Verification items for the finished model (mm, model axes). A direction names the side the tool comes from. Give positions to 0.01 mm unless a question says otherwise; leave off trailing zeros. Order: outer loops, then holes, each group sorted by start corner. A loop starts at its lowest first (then second) coordinate and runs counter-clockwise, first axis right, second up. Notation, with made-up numbers: (38, -4.5) -> (74, -4.5) arc R20 ccw to (74, 20.5) -> close; hole circle Ø2 at (26, 33). An arc over 180 degrees is marked (long way). Return JSON: item names as keys, results as strings. Group by question number.
(1) Release check for a two-part mould opening along Y. For faces 4 (the face through (-9.2, 0, 10.4)), 5 (the face through (0, 13.4, 12.8)), 6 (the face through (0.046, -17.387, 9.678)), 7 (the face through (0, 12, 6)) record: pulls with the +Y half, pulls with the -Y half, needs draft (parallel to the pull), parting line crosses it, or undercut.
(2) Cross-section at B-B on z = 4. Enter the section's corners in (x, y).
(3) Cross-section at C-C on y = -12.5. Enter the section's corners in (x, z), then the cut area to 3 significant figures.
(4) Depth check by flat-ended pin: pin 1 Ø1.1 at (x, y) = (-12.5, 0) entering from +Z; pin 2 Ø0.8 at (x, y) = (-1, -9) entering from +Z; pin 3 Ø5 at (y, z) = (13.5, 11) entering from -X. Enter the tip coordinate at first touch or a pass-through.
(5) Tool access check on faces 1 (the face through (11, 2.696, 5)), 2 (the face through (11, -2.696, 5)), 3 (the face through (-0.044, 10.565, 8.169)). Record the directions out of +Z, -Z, +X, -X, +Y, -Y that give a thin tool (end or side, any length) a straight path to the whole face; none if there is none.
(6) Cross-section at D-D on z = 7. State how many separate pieces and enclosed holes the cut face has, then the cut area to 3 significant figures.
(7) Thickness scan on line 1 along Y through (x, z) = (2, 9.5); line 2 along X through (y, z) = (1, 6.5); line 3 along Y through (x, z) = (15, 10.25). Record the ranges inside material, lowest first.
(8) Cross-section at A-A on z = 16. Enter the section's corners in (x, y).
from build123d import *

# Parameters (mm, degrees)
F2_R     = 0.5
F3_W     = 21.0270890966
F3_H     = 19.3190067075
F4_DEPTH = 25


with BuildPart() as f1:
    # F0 (on Front) → F1 (revolve)
    with BuildSketch(Plane.XZ):
        with BuildLine():
            Line((-20, 0), (0, 0))
            Line((0, 0), (0, 5))
            add(Edge.make_bspline(
                [(-9, 10.4), (-6.953539399, 4.2876302106), (0, 5)],
                knots=[3.4384028692, 3.4384028692, 3.4384028692, 4.8240705554, 4.8240705554, 4.8240705554], degree=2, weights=[1, 0.7694390741, 1]))
            Line((-9, 10.4), (-9.5, 10.4))
            Line((-9.5, 10.4), (-11.6, 6))
            Line((-11.6, 6), (-13.4, 6))
            Line((-13.4, 6), (-13.4, 20))
            Line((-13.4, 20), (-14.6, 20))
            Line((-14.6, 20), (-20, 0))
        make_face()
    revolve(axis=Axis((0, 0, 2.5), (0, 0, -1)))

    # F2
    f2_edges = [f1.edges().sort_by_distance(p)[0] for p in [
        (14.6, 0, 20),
        (13.4, 0, 20),
    ]]
    fillet(f2_edges, radius=F2_R)

    # F3 (on Top) → F4 (cut)
    with BuildSketch(Plane.XY):
        with Locations((-13.2951806299, 12.3554796446)):
            Rectangle(F3_W, F3_H)
        with Locations((13.2951806299, 12.3554796446)):
            Rectangle(F3_W, F3_H)
        with Locations((-13.2951806299, -12.3554796446)):
            Rectangle(F3_W, F3_H)
        with Locations((13.2951806299, -12.3554796446)):
            Rectangle(F3_W, F3_H)
    extrude(amount=F4_DEPTH, mode=Mode.SUBTRACT)


solid = f1.part
Verdict:
{
 "1": {"face 4": "needs draft", "face 5": "undercut", "face 6": "pulls with the -Y half", "face 7": "undercut"},
 "2": {"outline": "(-18.73, -2.7) -> (-2.78, -2.7) -> (-2.78, -18.71) arc R18.92 ccw to (2.78, -18.71) -> (2.78, -2.7) -> (18.73, -2.7) arc R18.92 ccw to (18.73, 2.7) -> (2.78, 2.7) -> (2.78, 18.71) arc R18.92 ccw to (-2.78, 18.71) -> (-2.78, 2.7) -> (-18.73, 2.7) arc R18.92 ccw to start"},
 "3": {"outline": "(-2.78, 0) -> (2.78, 0) -> (2.78, 6) -> (-2.78, 6) -> close", "area": "33.4 mm²"},
 "4": {"pin 1": "z = 6", "pin 2": "z = 10.4", "pin 3": "x = -2.78"},
 "5": {"face 1": "+Z, -Z, +X, +Y", "face 2": "+Z, -Z, +X, -Y", "face 3": "+Z"},
 "6": {"separate pieces": "8", "enclosed holes": "0", "area": "203 mm²"},
 "7": {"line 1": "-17.32 to -13.25, -9.73 to -8.4, 8.4 to 9.73, 13.25 to 17.32", "line 2": "-18.22 to -13.36, -11.32 to -5.92, 5.92 to 11.32, 13.36 to 18.22", "line 3": "-2.7 to 2.7"},
 "8": {"outline": "(-15.45, -2.7) -> (-13.13, -2.7) arc R13.4 cw to (-13.13, 2.7) -> (-15.45, 2.7) arc R15.68 ccw to start; (-2.78, -15.43) arc R15.68 ccw to (2.78, -15.43) -> (2.78, -13.11) arc R13.4 cw to (-2.78, -13.11) -> close; (-2.78, 13.11) arc R13.4 cw to (2.78, 13.11) -> (2.78, 15.43) arc R15.68 ccw to (-2.78, 15.43) -> close; (13.13, -2.7) -> (15.45, -2.7) arc R15.68 ccw to (15.45, 2.7) -> (13.13, 2.7) arc R13.4 cw to start"}
}
